For this review, use the dimensioned drawing (mm, ordinates from the lowest corner) and the shaded views. A direction names the side the tool comes from. Round coordinates to 2 decimals unless told otherwise and drop trailing zeros. Loops run counter-clockwise (first coordinate to the right, second up) from the corner with the lowest first, then second, coordinate; pieces in that order, holes last. Notation, with made-up numbers: (44, 70) - (57, 70) arc R17 ccw to (57, 89) - close; hole circle Ø10 at (25, 52.25). An arc over 180 degrees is marked (long way). Answer as CSV lines item,"result". Start each with the question number.
(1) Consider section A-A (y = 5.5). Give the boundary of the cut face in (x, z), and give its area (3 significant figures).
(2) Wall thickness on L1, parallel to X at y = 4.75, z = 0.25; L2, parallel to Y at x = 17.5, z = 1.65; L3, parallel to X at y = 7.25, z = 1.3: over which ranges is each line inside the solid? List them lowest first.
(3) Consider section C-C (z = 1.8). Give the boundary of the cut face in (x, y).
(4) Mouldability with a two-part tool opening along Y and no side actions: class the marked faces 1, 2 and 3 as released by +Y, released by -Y, zero draft, split by the parting line, or undercut.
(5) For the marked faces 4, 5, 6, 7 and 8, list the 3-axis set-ups (+Z, -Z, +X, -X, +Y, -Y) from which the entire face can be reached by the end or side of a thin tool; tool diameter is ignored.
(6) Consider section B-B (x = 17.5). Give the boundary of the cut face in (y, z).
(7) Consider section D-D (x = 13.25). Give the boundary of the cut face in (y, z).
(8) For P1, Ø0.6, axis at x = 18, z = 1.5, coming from the -Y side; P2, Ø1, axis at x = 1, z = 0.5, coming from the +Y side, all flat-tipped, find the tip position at first contact; note any pin that passes through.
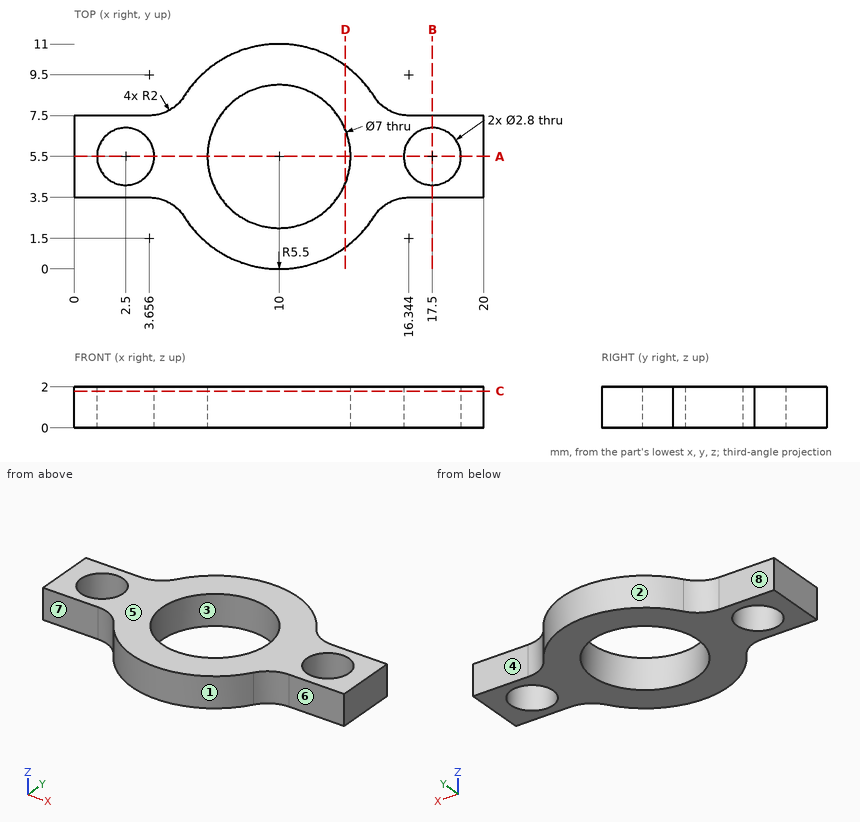
Determined:
1,outline,"(0, 0) - (1.1, 0) - (1.1, 2) - (0, 2) - close; (3.9, 0) - (6.5, 0) - (6.5, 2) - (3.9, 2) - close; (13.5, 0) - (16.1, 0) - (16.1, 2) - (13.5, 2) - close; (18.9, 0) - (20, 0) - (20, 2) - (18.9, 2) - close"
1,area,"14.8 mm^2"
2,L1,"x = 0 to 1.32, 3.68 to 6.58, 13.42 to 16.32, 18.68 to 20"
2,L2,"y = 3.5 to 4.1, 6.9 to 7.5"
2,L3,"x = 0 to 6.97, 13.03 to 20"
3,outline,"(0, 3.5) - (3.66, 3.5) arc R2 cw to (5.35, 2.57) arc R5.5 ccw to (14.65, 2.57) arc R2 cw to (16.34, 3.5) - (20, 3.5) - (20, 7.5) - (16.34, 7.5) arc R2 cw to (14.65, 8.43) arc R5.5 ccw to (5.35, 8.43) arc R2 cw to (3.66, 7.5) - (0, 7.5) - close; hole circle Ø2.8 at (2.5, 5.5); hole circle Ø7 at (10, 5.5); hole circle Ø2.8 at (17.5, 5.5)"
4,face 1,"released by -Y"
4,face 2,"released by +Y"
4,face 3,"undercut"
5,face 4,"+Z, -Z, +X, +Y"
5,face 5,"+Z, +X, -X, +Y, -Y"
5,face 6,"+Z, -Z, +X, -Y"
5,face 7,"+Z, -Z, -X, -Y"
5,face 8,"+Z, -Z, -X, +Y"
6,outline,"(3.5, 0) - (4.1, 0) - (4.1, 2) - (3.5, 2) - close; (6.9, 0) - (7.5, 0) - (7.5, 2) - (6.9, 2) - close"
7,outline,"(1.06, 0) - (4.2, 0) - (4.2, 2) - (1.06, 2) - close; (6.8, 0) - (9.94, 0) - (9.94, 2) - (6.8, 2) - close"
8,P1,"stops at y = 3.5"
8,P2,"stops at y = 7.5"
